from build123d import *

# Parameters (mm, degrees)
SKETCH_1_W         = 6.08
SKETCH_1_H         = 6.83
EXTRUDE_1_DEPTH    = 4.12
SKETCH_2_R         = 2.35
EXTRUDE_2_DEPTH    = 0.1
DOME_1_FACE_RADIUS = 2.35
DOME_1_HEIGHT      = 1.45
SKETCH_4_W         = 6.08
SKETCH_4_H         = 1
EXTRUDE_1_2_DEPTH  = 10


with BuildPart() as part:
    # 草图1 → Extrude 1 (new body)
    with BuildSketch(Plane.XY):
        Rectangle(SKETCH_1_W, SKETCH_1_H)
    extrude(amount=EXTRUDE_1_DEPTH)

    # 草图2 → 拉伸2 (add)
    with BuildSketch(Plane(origin=(0, 0, 0), x_dir=(-1, 0, 0), z_dir=(0, 0, -1))):
        with Locations(Location((0, 0.565, 0), (0, 0, 180))):
            Circle(SKETCH_2_R)
    extrude(amount=EXTRUDE_2_DEPTH)

    # 圆顶1: a dome of height H over a round flat face of radius A is a cap of a sphere of radius (A * A + H * H) / (2 * H)
    dome_1_r = (DOME_1_FACE_RADIUS * DOME_1_FACE_RADIUS + DOME_1_HEIGHT * DOME_1_HEIGHT) / (2 * DOME_1_HEIGHT)
    dome_1_base = Plane((0, 0.565, -0.1), z_dir=(0, 0, -1))
    with Locations(dome_1_base.offset(DOME_1_HEIGHT - dome_1_r)):
        dome_1_ball = Sphere(dome_1_r, mode=Mode.PRIVATE)
    add(split(dome_1_ball, bisect_by=dome_1_base, keep=Keep.TOP, mode=Mode.PRIVATE))

    # 草图4 → Extrude 1 2 (add)
    with BuildSketch(Plane.XZ.offset(3.415)):
        with Locations((0, 3.12)):
            Rectangle(SKETCH_4_W, SKETCH_4_H)
    extrude(amount=EXTRUDE_1_2_DEPTH)


solid = part.part
Geometry check sheet. Reference: the model listing, model coordinates, mm. A direction names the side the tool comes from. Round coordinates to 2 decimals unless told otherwise and drop trailing zeros. Loops run counter-clockwise (first coordinate to the right, second up) from the corner with the lowest first, then second, coordinate; pieces in that order, holes last. Notation, with made-up numbers: (54.25, 62) -> (70.25, 62) arc R25 cw to (70.25, 101) -> close; hole circle Ø2 at (-40, -29). An arc over 180 degrees is marked (long way). Answer as a JSON object with one key per item and string values. Group by question number.
Item 1: Cross-section at B-B, the plane y = -11.75. Record the cut outline in (x, z), plus the area to 3 significant figures.
Item 2: Cross-section at D-D, the plane x = 1.25. Record the cut outline in (y, z) (3 decimals).
Item 3: Set-up check for faces 1 (the face through (3.04, -1, 2)), 2 (the face through (0, -2, 0)), 3 (the face through (0, -8, 3.62)), 4 (the face through (0, -3.415, 1)): record each of +Z, -Z, +X, -X, +Y, -Y from which the full face is reachable in a straight line by a thin tool's end or side.
Item 4: Cross-section at C-C, the plane z = 1.7. Record the cut outline in (x, y) (3 decimals), plus the area to 3 significant figures.
Item 5: Cross-section at A-A, the plane x = 0. Record the cut outline in (y, z) (3 decimals), plus the area to 3 significant figures.
Item 6: Thickness scan on line 1 along Z through (x, y) = (-2, -1.75); line 2 along Y through (x, z) = (0.25, 0.7) (3 decimals); line 3 along Z through (x, y) = (-1, -9.5). Record the ranges inside material, lowest first.
Item 7: Depth check by flat-ended pin: pin 1 Ø1.5 at (x, z) = (2, -0.5) entering from -Y (3 decimals); pin 2 Ø1 at (x, y) = (1, -4.5) entering from +Z; pin 3 Ø1.8 at (x, y) = (-0.5, -10.5) entering from -Z. Enter the tip coordinate at first touch or a pass-through.
Determined:
{
 "1": {"outline": "(-3.04, 2.62) -> (3.04, 2.62) -> (3.04, 3.62) -> (-3.04, 3.62) -> close", "area": "6.08 mm²"},
 "2": {"outline": "(-13.415, 2.62) -> (-3.415, 2.62) -> (-3.415, 0) -> (-1.425, 0) -> (-1.425, -0.1) arc R2.313 ccw to (2.555, -0.1) -> (2.555, 0) -> (3.415, 0) -> (3.415, 4.12) -> (-3.415, 4.12) -> (-3.415, 3.62) -> (-13.415, 3.62) -> close"},
 "3": {"face 1": "+Z, -Z, +X, +Y, -Y", "face 2": "-Z", "face 3": "+Z, +X, -X, -Y", "face 4": "-Z, +X, -X, -Y"},
 "4": {"outline": "(-3.04, -3.415) -> (3.04, -3.415) -> (3.04, 3.415) -> (-3.04, 3.415) -> close", "area": "41.5 mm²"},
 "5": {"outline": "(-13.415, 2.62) -> (-3.415, 2.62) -> (-3.415, 0) -> (-1.785, 0) -> (-1.785, -0.1) arc R2.629 ccw to (2.915, -0.1) -> (2.915, 0) -> (3.415, 0) -> (3.415, 4.12) -> (-3.415, 4.12) -> (-3.415, 3.62) -> (-13.415, 3.62) -> close", "area": "43.5 mm²"},
 "6": {"line 1": "z = 0 to 4.12", "line 2": "y = -3.415 to 3.415", "line 3": "z = 2.62 to 3.62"},
 "7": {"pin 1": "stops at y = -3.415", "pin 2": "stops at z = 3.62", "pin 3": "stops at z = 2.62"}
}
